Read the model definition and answer for the solid it produces. Units are mm, in the model's axes. A direction names the side the tool comes from. Coordinates: 2 decimals unless noted, no trailing zeros. Write each loop counter-clockwise with the first axis right and the second up, starting at its lowest first coordinate (ties: lowest second). Pieces come first, ordered by that corner, then holes. Notation, with made-up numbers: (50.5, 60.5) -> (63.5, 60.5) arc R27 ccw to (63.5, 78.5) -> close; hole circle Ø4 at (-33.5, 60). An arc over 180 degrees is marked (long way). Answer in a Markdown table with one row per item. Add a question column.
Item 1: For a pull along X with two mould halves and no side action, classify faces 1 (the face through (58, 35, 1)), 2 (the face through (61, 17, 1)), 3 (the face through (60.98, 31.97, 4.89)), 4 (the face through (60.98, 1.97, 4.89)) as +X half, -X half, draft (parallel to the pull), parting line (faces both ways), or undercut.
Item 2: Section C-C on z = 1.5 is taken. Write down the section's boundary in (x, y), then the cut area to 3 significant figures.
Item 3: Straight lines are drawn through the part: line 1 (Z direction, x = 59.5, y = 33.1); line 2 (Z direction, x = 53.5, y = 12); line 3 (X direction, y = 8.5, z = 6). For each, find the intervals that lie inside material, in ascending order. Write a range as from..to.
Item 4: Section D-D on x = 35 is taken. Write down the section's boundary in (y, z).
Item 5: Given pin 1 Ø1 at (y, z) = (2, 6.5) entering from +X; pin 2 Ø2.5 at (y, z) = (2.5, 3.5) entering from -X; pin 3 Ø3.5 at (x, y) = (59, 36) entering from +Z; pin 4 Ø2.5 at (x, z) = (59.5, 5.5) entering from +Y, each flat-ended and moving along its own axis, determine where each tip first touches the part or whether it passes through.
Item 6: Section A-A on x = 3 is taken. Write down the section's boundary in (y, z), then the cut area to 3 significant figures.
Item 7: Which of the six approach directions +Z, -Z, +X, -X, +Y, -Y give full straight-line access (tool end or side, diameter ignored) to faces 5 (the face through (60, 35, 2.5)), 6 (the face through (58, -1, 1)), 7 (the face through (60, -1, 2.5)), 8 (the face through (4.13, 16.76, 7.27)), 9 (the face through (56.5, 2, 4))?
Item 8: Section B-B on y = 8.5 is taken. Write down the section's boundary in (x, z), then the cut area to 3 significant figures.
```python
from build123d import *

# Parameters (mm, degrees)
SKETCH_1_W                  = 60
SKETCH_1_H                  = 34
EXTRUDE_1_DEPTH             = 2.5
SKETCH_3_R                  = 3
SKETCH_3_R_2                = 1.6
EXTRUDE_2_DEPTH             = 4
PATTERN_LINEAR_1_COUNT      = 2
PATTERN_LINEAR_1_PITCH      = 56.5
PATTERN_LINEAR_1_COUNT_DIR2 = 2
PATTERN_LINEAR_1_PITCH_DIR2 = 30
SKETCH_5_W                  = 2.5
SKETCH_5_H                  = 34
EXTRUDE_3_DEPTH             = 4
SKETCH_6_W                  = 2.5
SKETCH_6_H                  = 34
EXTRUDE_4_DEPTH             = 4
CUT_EXTRUDE_1_DEPTH         = 73.9674585
EXTRUDE_13_REACH            = 73.192
SKETCH_8_R                  = 1.6
CUT_EXTRUDE_2_DEPTH         = 73.9674585
EXTRUDE_START               = -34
EXTRUDE_14_DEPTH            = 34
SKETCH_10_W                 = 1.5
SKETCH_10_H                 = 2.5
CUT_EXTRUDE_3_DEPTH         = 34
CUT_EXTRUDE_4_DEPTH         = 72.655425475
CUT_EXTRUDE_4_DEPTH_BACK    = 72.655425475
EXTRUDE_16_DEPTH            = 3
EXTRUDE_17_DEPTH            = 3
SKETCH_15_R                 = 2.1
CUT_EXTRUDE_6_DEPTH         = 74.126602547
EXTRUDE_18_DEPTH            = 34
FILLET_1_R                  = 5


# Read off the part's stored shape, not the designer's step: 凸台-拉伸18
with BuildPart() as part:
    # 草图1 → 凸台-拉伸1 (new body)
    with BuildSketch(Plane.XY):
        with Locations((30, 17)):
            Rectangle(SKETCH_1_W, SKETCH_1_H)
    extrude(amount=EXTRUDE_1_DEPTH)

    # 草图3 → 凸台-拉伸2 (add)
    # profile 1 of 3: a face of its own
    with BuildSketch(Plane.XZ):
        with BuildLine():
            Line((6, 2.5), (6, 5.5))
            ThreePointArc((6, 5.5), (5.121320344, 3.378679656), (3, 2.5))
            Line((3, 2.5), (6, 2.5))
        make_face()
    # profile 2 of 3: a face of its own
    with BuildSketch(Plane.XZ):
        with BuildLine():
            ThreePointArc((3, 2.5), (0.878679656, 3.378679656), (0, 5.5))
            Line((0, 5.5), (0, 2.5))
            Line((0, 2.5), (3, 2.5))
        make_face()
    # profile 3 of 3: a face of its own
    with BuildSketch(Plane.XZ):
        with Locations((3, 5.5)):
            Circle(SKETCH_3_R)
        with Locations((3, 5.5)):
            Circle(SKETCH_3_R_2, mode=Mode.SUBTRACT)
    extrude_2 = extrude(amount=-EXTRUDE_2_DEPTH)

    # 阵列(线性)1: Extrude 2 2 × 2
    with Locations(*[(i * PATTERN_LINEAR_1_PITCH, j * PATTERN_LINEAR_1_PITCH_DIR2, 0) for i in range(PATTERN_LINEAR_1_COUNT) for j in range(PATTERN_LINEAR_1_COUNT_DIR2) if (i, j) != (0, 0)]):
        add(extrude_2)

    # 草图5 → 凸台-拉伸3 (add)
    with BuildSketch(Plane.ZY):
        with Locations((1.25, 17)):
            Rectangle(SKETCH_5_W, SKETCH_5_H)
    extrude(amount=EXTRUDE_3_DEPTH)

    # 草图6 → 凸台-拉伸4 (add)
    with BuildSketch(Plane(origin=(60, 0, 0), x_dir=(0, 0, -1), z_dir=(1, 0, 0))):
        with Locations((-1.25, 17)):
            Rectangle(SKETCH_6_W, SKETCH_6_H)
    extrude(amount=EXTRUDE_4_DEPTH)

    # 草图7 → 切除-拉伸1 (cut, through all)
    with BuildSketch(Plane(origin=(0, 34, 0), x_dir=(1, 0, 0), z_dir=(0, 1, 0))):
        with BuildLine():
            ThreePointArc((0, -5.5), (0.878679656, -3.378679656), (3, -2.5))
            Line((3, -2.5), (3, 0))
            Line((3, 0), (-4, 0))
            Line((-4, 0), (-4, -2.5))
            Line((-4, -2.5), (0, -2.5))
            Line((0, -2.5), (0, -5.5))
        make_face()
    extrude(amount=-CUT_EXTRUDE_1_DEPTH, mode=Mode.SUBTRACT)

    # 草图8 → 凸台-拉伸13 (add, up to next)
    with BuildSketch(Plane(origin=(0, 4, 0), x_dir=(1, 0, 0), z_dir=(0, 1, 0)), mode=Mode.PRIVATE) as extrude_13_sk1:
        with BuildLine():
            ThreePointArc((3, -2.5), (0.878679656, -7.621320344), (6, -5.5))
            ThreePointArc((6, -5.5), (5.121320344, -3.378679656), (3, -2.5))
        make_face()
        with Locations((3, -5.5)):
            Circle(SKETCH_8_R, mode=Mode.SUBTRACT)
    extrude_13_tool1 = extrude(extrude_13_sk1.sketch, amount=EXTRUDE_13_REACH, mode=Mode.PRIVATE) - part.part
    # 草图8 → 凸台-拉伸13 (add, up to next)
    with BuildSketch(Plane(origin=(0, 4, 0), x_dir=(1, 0, 0), z_dir=(0, 1, 0)), mode=Mode.PRIVATE) as extrude_13_sk2:
        with BuildLine():
            ThreePointArc((3, -2.5), (5.121320344, -3.378679656), (6, -5.5))
            Line((6, -5.5), (6, -2.5))
            Line((6, -2.5), (3, -2.5))
        make_face()
    extrude_13_tool2 = extrude(extrude_13_sk2.sketch, amount=EXTRUDE_13_REACH, mode=Mode.PRIVATE) - part.part
    add(extrude_13_tool1.solids().sort_by_distance((5.06132, 4, 3.43868))[0])
    add(extrude_13_tool2.solids().sort_by_distance((5.329896, 4, 3.170104))[0])

    # 草图9 → 切除-拉伸2 (cut, through all)
    with BuildSketch(Plane(origin=(0, 34, 0), x_dir=(1, 0, 0), z_dir=(0, 1, 0))):
        Polygon((3, 0), (3, -2.035898385), (6.526279442, 0), align=None)
    extrude(amount=-CUT_EXTRUDE_2_DEPTH, mode=Mode.SUBTRACT)

    # 草图9<3> → 凸台-拉伸14 (add)
    with BuildSketch(Plane(origin=(0, 34, 0), x_dir=(1, 0, 0), z_dir=(0, 1, 0)).offset(EXTRUDE_START)):
        Polygon((6, -2.5), (6, -3.190598923), (7.196152423, -2.5), align=None)
        with BuildLine():
            Line((3, -2.035898385), (1.5, -2.901923789))
            ThreePointArc((1.5, -2.901923789), (2.223542865, -2.602222521), (3, -2.5))
            Line((3, -2.5), (3, -2.035898385))
        make_face()
    extrude(amount=EXTRUDE_14_DEPTH)

    # 草图10 → 切除-拉伸3 (cut)
    with BuildSketch(Plane(origin=(0, 34, 0), x_dir=(1, 0, 0), z_dir=(0, 1, 0))):
        with Locations((63.25, -1.25)):
            Rectangle(SKETCH_10_W, SKETCH_10_H)
    extrude(amount=-CUT_EXTRUDE_3_DEPTH, mode=Mode.SUBTRACT)

    # 草图11 → 切除-拉伸4 (cut, two sides: drawn at the far end of the back side and taken through both)
    with BuildSketch(Plane(origin=(0, 34, 0), x_dir=(1, 0, 0), z_dir=(0, 1, 0)).offset(-CUT_EXTRUDE_4_DEPTH_BACK)):
        Polygon((60, 0), (62.5, -2.5), (62.5, 0), align=None)
    extrude(amount=CUT_EXTRUDE_4_DEPTH + CUT_EXTRUDE_4_DEPTH_BACK, mode=Mode.SUBTRACT)

    # 草图13 → 凸台-拉伸16 (add)
    with BuildSketch(Plane(origin=(0, 34, 0), x_dir=(1, 0, 0), z_dir=(0, 1, 0))):
        Polygon((62.5, -2.5), (58, -2.5), (58, 0), (60, 0), align=None)
    extrude(amount=EXTRUDE_16_DEPTH)

    # 草图14 → 凸台-拉伸17 (add)
    with BuildSketch(Plane.XZ):
        Polygon((62.5, 2.5), (60, 0), (58, 0), (58, 2.5), align=None)
    extrude(amount=EXTRUDE_17_DEPTH)

    # 草图15 → 切除-拉伸6 (cut, through all)
    with BuildSketch(Plane.XZ):
        with Locations((3, 5.5)):
            Circle(SKETCH_15_R)
    extrude(amount=-CUT_EXTRUDE_6_DEPTH, mode=Mode.SUBTRACT)

    # 凸台-拉伸18 outline → 凸台-拉伸18 (add)
    with BuildSketch(Plane(origin=(0, 0, 0), x_dir=(-1, 0, 0), z_dir=(0, -1, 0)).offset(EXTRUDE_START)):
        with BuildLine():
            Line((-7.196152423, -2.5), (-6.5, -5.5))
            ThreePointArc((-6.5, -5.5), (-1.117959969, -8.450919402), (-1.524042675, -2.32642946))
            Line((-1.524042675, -2.32642946), (-6.526279442, 0))
            Line((-6.526279442, 0), (-1.5, -2.901923789))
            ThreePointArc((-1.5, -2.901923789), (-1.5, -8.098076211), (-6, -5.5))
            Line((-6, -5.5), (-6, -3.190598923))
            Line((-6, -3.190598923), (-7.196152423, -2.5))
        make_face()
    extrude(amount=EXTRUDE_18_DEPTH)

    # 圆角1
    # the kernel refuses this fillet: 5 mm, written as the material it adds along each edge
    with BuildSketch(Plane(origin=(7.196152423, 0, 2.5), x_dir=(1, 0, 0), z_dir=(0, 1, 0))) as fillet_1_piece_1:
        with BuildLine():
            CenterArc((3.886423272, -5), FILLET_1_R, 90, 66.421821522)
            Line((-0.696152423, -3), (-0.787803937, -2.96))
            ThreePointArc((-0.787803937, -2.96), (-0.445487906, -1.477395538), (-0.097411695, 0.022604462))
            Line((-0.097411695, 0.022604462), (0, 0.1))
            Line((0, 0.1), (3.886423272, 0.1))
            Line((3.886423272, 0.1), (3.886423272, 0))
        make_face()
    extrude(amount=34)


solid = part.part
```
Results below:
| question | item | result |
|---|---|---|
| 1 | face 1 | -X half |
| 1 | face 2 | +X half |
| 1 | face 3 | undercut |
| 1 | face 4 | undercut |
| 2 | outline | (3.3, 0) -> (58, 0) -> (58, -3) -> (61.5, -3) -> (61.5, 37) -> (58, 37) -> (58, 34) -> (3.3, 34) -> close |
| 2 | area | 2,000 mm2 |
| 3 | line 1 | z = 0..3.9, 7.1..8.5 |
| 3 | line 2 | z = 0..2.5 |
| 3 | line 3 | x = -0.46..0.96, 5.04..6.46 |
| 4 | outline | (0, 0) -> (34, 0) -> (34, 2.5) -> (0, 2.5) -> close |
| 5 | pin 1 | stops at x = 62.46 |
| 5 | pin 2 | stops at x = -0.42 |
| 5 | pin 3 | stops at z = 2.5 |
| 5 | pin 4 | passes through |
| 6 | outline | (0, 1.64) -> (34, 1.64) -> (34, 3.4) -> (0, 3.4) -> close; (0, 7.6) -> (34, 7.6) -> (34, 9) -> (0, 9) -> close |
| 6 | area | 107 mm2 |
| 7 | face 5 | +Z, +X, -X, +Y |
| 7 | face 6 | +Z, -Z, -X, -Y |
| 7 | face 7 | +Z, +X, -X, -Y |
| 7 | face 8 | +Y, -Y |
| 7 | face 9 | +Z, +Y, -Y |
| 8 | outline | (1.52, 2.33) -> (6.53, 0) -> (60, 0) -> (62.5, 2.5) -> (11.08, 2.5) arc R5 cw to (6.5, 5.5) arc R3.5 ccw (long way) to start; hole circle Ø4.2 at (3, 5.5) |
| 8 | area | 172 mm2 |
